from build123d import *

# Parameters (mm, degrees)
SKETCH_1_R      = 27.5
SKETCH_1_R_2    = 2
EXTRUDE_1_DEPTH = 8
SKETCH_2_R      = 5
EXTRUDE_2_DEPTH = 182


with BuildPart() as part:
    # 草图1 → 凸台-拉伸1 (new body)
    with BuildSketch(Plane.XY):
        Circle(SKETCH_1_R)
        with Locations((-17.25, 0)):
            Circle(SKETCH_1_R_2, mode=Mode.SUBTRACT)
        with Locations((-8.625, 14.938938215)):
            Circle(SKETCH_1_R_2, mode=Mode.SUBTRACT)
        with Locations((8.625, 14.938938215)):
            Circle(SKETCH_1_R_2, mode=Mode.SUBTRACT)
        with Locations((17.25, 0)):
            Circle(SKETCH_1_R_2, mode=Mode.SUBTRACT)
        with Locations((8.625, -14.938938215)):
            Circle(SKETCH_1_R_2, mode=Mode.SUBTRACT)
        with Locations((-8.625, -14.938938215)):
            Circle(SKETCH_1_R_2, mode=Mode.SUBTRACT)
    extrude(amount=EXTRUDE_1_DEPTH)

    # 草图2 → 凸台-拉伸2 (add)
    with BuildSketch(Plane.XY.offset(8)):
        Circle(SKETCH_2_R)
    extrude(amount=EXTRUDE_2_DEPTH)


solid = part.part
Can you work these out from the model? Positions are in its coordinate system, mm. A direction names the side the tool comes from. Coordinates: 2 decimals unless noted, no trailing zeros. Write each loop counter-clockwise with the first axis right and the second up, starting at its lowest first coordinate (ties: lowest second). Pieces come first, ordered by that corner, then holes. Notation, with made-up numbers: M -27.5,74.5 L -19.5,74.5 A33 ccw -19.5,104.5 Z; hole C 67.5,69.5 d11. An arc over 180 degrees is marked long. Use one line per item in the form item = value.
Q1. I need wall thicknesses on line 1 along Z through (x, y) = (-12.5, -20); line 2 along X through (y, z) = (-0.5, 112); line 3 along Y through (x, z) = (0, 72.5). Which ranges of each line are inside material? Lowest first, please. Write a range as from..to.
Model answer:
line_1 = 0..8
line_2 = -4.97..4.97
line_3 = -5..5
Q2. If we section it at C-C (x = 0): Write out the boundary of the cut face in (y, z), then the cut area to 3 significant figures.
Model answer:
outline = M -27.5,0 L 27.5,0 L 27.5,8 L 5,8 L 5,190 L -5,190 L -5,8 L -27.5,8 Z
area = 2,260 mm^2
Q3. If we section it at D-D (z = 87): Write out the boundary of the cut face in (x, y).
Model answer:
outline = C 0,0 d10
Q4. We'd pull the mould along X, two halves only. Please class faces 1 (the cylindrical face through (-8.885, -12.956, 3.944)), 2 (the cylindrical face through (-5.961, -26.846, 3.944)), 3 (the cylindrical face through (8.36, 16.92, 3.94)), 4 (the flat face through (0, 0, 0)): +X half, -X half, draft (parallel to the pull), parting line (faces both ways), or undercut.
Model answer:
face_1 = undercut
face_2 = parting line
face_3 = undercut
face_4 = draft
Q5. For faces 5 (the cylindrical face through (-8.89, 16.92, 3.94)), 6 (the cylindrical face through (-1.08, -4.88, 97.73)), which set-ups out of +Z, -Z, +X, -X, +Y, -Y let a thin tool reach every point of the face, with its end or its side?
Model answer:
face_5 = +Z, -Z
face_6 = +Z
Q6. If we section it at B-B (x = 17.25): Write out the boundary of the cut face in (y, z).
Model answer:
outline = M -21.42,0 L -2,0 L -2,8 L -21.42,8 Z; M 2,0 L 21.42,0 L 21.42,8 L 2,8 Z
Q7. For P1, Ø2.5, axis at x = -8.62, y = 14.94, coming from the +Z side; P2, Ø2, axis at x = -4.5, z = 157.5, coming from the -Y side, each with a flat end and sliding along its axis, tell me the tip position at first contact or that it passes through.
Model answer:
P1 = through
P2 = -3.57
Q8. If we section it at A-A (y = 0): Write out the boundary of the cut face in (x, z), then the cut area to 3 significant figures.
Model answer:
outline = M -27.5,0 L -19.25,0 L -19.25,8 L -27.5,8 Z; M -15.25,0 L 15.25,0 L 15.25,8 L 5,8 L 5,190 L -5,190 L -5,8 L -15.25,8 Z; M 19.25,0 L 27.5,0 L 27.5,8 L 19.25,8 Z
area = 2,200 mm^2
